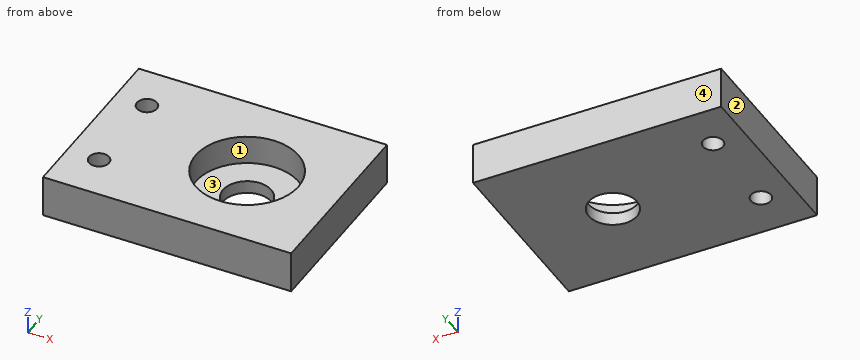
from build123d import *

# Parameters (mm, degrees)
SKETCH1_W                        = 77.3
SKETCH1_H                        = 57.3
BOSS_EXTRUDE1_DEPTH              = 13
TAP_DRILL_FOR_M6_HELICOIL1_D     = 6.25
TAP_DRILL_FOR_M6_HELICOIL1_DEPTH = 20
TAP_DRILL_FOR_M6_HELICOIL1_TIP   = 1.877689434
SKETCH2_R                        = 16
CUT_EXTRUDE1_DEPTH               = 9
SKETCH6_R                        = 7.5
CUT_EXTRUDE2_DEPTH               = 9


with BuildPart() as part:
    # Sketch1 → Boss-Extrude1 (new body)
    with BuildSketch(Plane.XY):
        Rectangle(SKETCH1_W, SKETCH1_H)
    extrude(amount=BOSS_EXTRUDE1_DEPTH)

    # Tap Drill for M6 Helicoil1
    with Locations(Plane(origin=(-28.65, 14.325, 13), x_dir=(1, 0, 0), z_dir=(0, 0, 1))):
        with Locations((0, 0), (0, -28.65)):
            Hole(TAP_DRILL_FOR_M6_HELICOIL1_D / 2, depth=TAP_DRILL_FOR_M6_HELICOIL1_DEPTH)
            with Locations((0, 0, -(TAP_DRILL_FOR_M6_HELICOIL1_DEPTH + TAP_DRILL_FOR_M6_HELICOIL1_TIP / 2))):  # 118° drill point
                Cone(0, TAP_DRILL_FOR_M6_HELICOIL1_D / 2, TAP_DRILL_FOR_M6_HELICOIL1_TIP, mode=Mode.SUBTRACT)

    # Sketch2 → Cut-Extrude1 (cut)
    with BuildSketch(Plane.XY.offset(13)):
        with Locations((10, 0)):
            Circle(SKETCH2_R)
    extrude(amount=-CUT_EXTRUDE1_DEPTH, mode=Mode.SUBTRACT)

    # Sketch6 → Cut-Extrude2 (cut)
    with BuildSketch(Plane.XY.offset(4)):
        with Locations((10, 0)):
            Circle(SKETCH6_R)
    extrude(amount=-CUT_EXTRUDE2_DEPTH, mode=Mode.SUBTRACT)


solid = part.part
The listing builds one solid part. Answer for the finished solid, in the listing's coordinates (mm). Face numbers are marked on the shaded views. Coordinates: 2 decimals unless noted, no trailing zeros. Order: outer loops, then holes, each group sorted by start corner. A loop starts at its lowest first (then second) coordinate and runs counter-clockwise, first axis right, second up. Notation, with made-up numbers: (25.5, 40.5) -> (78.5, 40.5) arc R22 cw to (78.5, 62.5) -> close; hole circle Ø1 at (76, -19). An arc over 180 degrees is marked (long way). Answer in a Markdown table with one row per item. Add a question column.
Item 1: Find section C-C (x = 10). Write down the section's boundary in (y, z).
Item 2: Find the intervals of material crossed by L1, parallel to Y at x = -28.65, z = 2.75; L2, parallel to Y at x = -26, z = 2.75; L3, parallel to X at y = 12, z = 8, in increasing order. Write a range as from..to.
Item 3: Determine the mould class of the marked faces 1, 2, 3 and 4 for opening direction Y: +Y half, -Y half, draft (parallel to the pull), parting line (faces both ways), or undercut.
Item 4: Find section A-A (y = 0). Write down the section's boundary in (x, z).
Item 5: This flat-tipped pin is pushed along its axis until it touches: P1, Ø17, axis at x = 10, y = 0, coming from the +Z side. Where does it stop, or does it pass through?
Item 6: Find section B-B (x = -28.65). Write down the section's boundary in (y, z), then the cut area to 3 significant figures.
Item 7: Find section D-D (z = 9.25). Write down the section's boundary in (x, y) (3 decimals), then the cut area to 3 significant figures.
Result set:
| question | item | result |
|---|---|---|
| 1 | outline | (-28.65, 0) -> (-7.5, 0) -> (-7.5, 4) -> (-16, 4) -> (-16, 13) -> (-28.65, 13) -> close; (7.5, 0) -> (28.65, 0) -> (28.65, 13) -> (16, 13) -> (16, 4) -> (7.5, 4) -> close |
| 2 | L1 | y = -28.65..-17.45, -11.2..11.2, 17.45..28.65 |
| 2 | L2 | y = -28.65..-15.98, -12.67..12.67, 15.98..28.65 |
| 2 | L3 | x = -38.65..-30.74, -26.56..-0.58, 20.58..38.65 |
| 3 | face 1 | undercut |
| 3 | face 2 | draft |
| 3 | face 3 | undercut |
| 3 | face 4 | +Y half |
| 4 | outline | (-38.65, 0) -> (2.5, 0) -> (2.5, 4) -> (-6, 4) -> (-6, 13) -> (-38.65, 13) -> close; (17.5, 0) -> (38.65, 0) -> (38.65, 13) -> (26, 13) -> (26, 4) -> (17.5, 4) -> close |
| 5 | P1 | stops at z = 4 |
| 6 | outline | (-28.65, 0) -> (-17.45, 0) -> (-17.45, 13) -> (-28.65, 13) -> close; (-11.2, 0) -> (11.2, 0) -> (11.2, 13) -> (-11.2, 13) -> close; (17.45, 0) -> (28.65, 0) -> (28.65, 13) -> (17.45, 13) -> close |
| 6 | area | 582 mm² |
| 7 | outline | (-38.65, -28.65) -> (38.65, -28.65) -> (38.65, 28.65) -> (-38.65, 28.65) -> close; hole circle Ø6.25 at (-28.65, -14.325); hole circle Ø6.25 at (-28.65, 14.325); hole circle Ø32 at (10, 0) |
| 7 | area | 3,560 mm² |
